from build123d import *

# Parameters (mm, degrees)
SKETCH2_R           = 2
BOSS_EXTRUDE2_DEPTH = 3.175


with BuildPart() as part:
    # Sketch2 → Boss-Extrude2 (new body)
    with BuildSketch(Plane.XY):
        with BuildLine():
            ThreePointArc((9.456794765, 7.302125235), (10.51328966, 8.920913041), (10.82870315, 10.828049574))
            ThreePointArc((10.82870315, 10.828049574), (8.921045244, 10.513465667), (7.301533296, 9.457386704))
            ThreePointArc((7.301533296, 9.457386704), (5.308889045, 9.194845217), (4.539183834, 11.051485471))
            ThreePointArc((4.539183834, 11.051485471), (4.64471403, 12.981928422), (3.964051405, 14.791471183))
            ThreePointArc((3.964051405, 14.791471183), (2.469674584, 13.565372247), (1.59532555, 11.841424903))
            ThreePointArc((1.59532555, 11.841424903), (0.000409384, 10.617090374), (-1.594506782, 11.841424903))
            ThreePointArc((-1.594506782, 11.841424903), (-2.468043552, 13.565085875), (-3.961395494, 14.791451895))
            ThreePointArc((-3.961395494, 14.791451895), (-4.64300424, 12.982116437), (-4.538365066, 11.051485471))
            ThreePointArc((-4.538365066, 11.051485471), (-5.308070277, 9.194845217), (-7.300714528, 9.457386704))
            ThreePointArc((-7.300714528, 9.457386704), (-8.919846484, 10.513683908), (-10.827230806, 10.82870315))
            ThreePointArc((-10.827230806, 10.82870315), (-10.512252617, 8.921293027), (-9.455975997, 7.302125235))
            ThreePointArc((-9.455975997, 7.302125235), (-9.19343451, 5.309480984), (-11.050074764, 4.539775774))
            ThreePointArc((-11.050074764, 4.539775774), (-12.980517715, 4.64530597), (-14.790060475, 3.964643344))
            ThreePointArc((-14.790060475, 3.964643344), (-13.56396154, 2.470266524), (-11.840014195, 1.595917489))
            ThreePointArc((-11.840014195, 1.595917489), (-10.615679667, 0.001001323), (-11.840014195, -1.593914842))
            ThreePointArc((-11.840014195, -1.593914842), (-13.563675168, -2.467451613), (-14.790041187, -3.960803554))
            ThreePointArc((-14.790041187, -3.960803554), (-12.980705729, -4.6424123), (-11.050074764, -4.537773127))
            ThreePointArc((-11.050074764, -4.537773127), (-9.19343451, -5.307478337), (-9.455975997, -7.300122588))
            ThreePointArc((-9.455975997, -7.300122588), (-10.512273201, -8.919254544), (-10.827292443, -10.826638866))
            ThreePointArc((-10.827292443, -10.826638866), (-8.91988232, -10.511660678), (-7.300714528, -9.455384057))
            ThreePointArc((-7.300714528, -9.455384057), (-5.308070277, -9.19284257), (-4.538365066, -11.049482824))
            ThreePointArc((-4.538365066, -11.049482824), (-4.643895262, -12.979925775), (-3.963232637, -14.789468536))
            ThreePointArc((-3.963232637, -14.789468536), (-2.468855816, -13.5633696), (-1.594506782, -11.839422256))
            ThreePointArc((-1.594506782, -11.839422256), (0.000409384, -10.615087727), (1.59532555, -11.839422256))
            ThreePointArc((1.59532555, -11.839422256), (2.46886232, -13.563083228), (3.962214262, -14.789449248))
            ThreePointArc((3.962214262, -14.789449248), (4.643823008, -12.98011379), (4.539183834, -11.049482824))
            ThreePointArc((4.539183834, -11.049482824), (5.308889045, -9.19284257), (7.301533296, -9.455384057))
            ThreePointArc((7.301533296, -9.455384057), (8.920665252, -10.511681261), (10.828049574, -10.826700503))
            ThreePointArc((10.828049574, -10.826700503), (10.513071385, -8.91929038), (9.456794765, -7.300122588))
            ThreePointArc((9.456794765, -7.300122588), (9.194253278, -5.307478337), (11.050893532, -4.537773127))
            ThreePointArc((11.050893532, -4.537773127), (12.981336483, -4.643303323), (14.790879243, -3.962640697))
            ThreePointArc((14.790879243, -3.962640697), (13.564780308, -2.468263877), (11.840832964, -1.593914842))
            ThreePointArc((11.840832964, -1.593914842), (10.617899153, 0.000932392), (11.841424903, 1.59532555))
            ThreePointArc((11.841424903, 1.59532555), (13.565085875, 2.46886232), (14.791451895, 3.962214262))
            ThreePointArc((14.791451895, 3.962214262), (12.982116437, 4.643823008), (11.051485471, 4.539183834))
            ThreePointArc((11.051485471, 4.539183834), (9.193282623, 5.308357949), (9.456794765, 7.302125235))
        make_face()
        Circle(SKETCH2_R, mode=Mode.SUBTRACT)
    extrude(amount=BOSS_EXTRUDE2_DEPTH)


solid = part.part
Verification items for the finished model (mm, model axes). A direction names the side the tool comes from. Give positions to 0.01 mm unless a question says otherwise; leave off trailing zeros. Write each loop counter-clockwise with the first axis right and the second up, starting at its lowest first coordinate (ties: lowest second). Pieces come first, ordered by that corner, then holes. Notation, with made-up numbers: M 33,72.5 L 58,72.5 A13 ccw 58,88.5 Z; hole C -21.5,84.5 d2. An arc over 180 degrees is marked long. Put each result on its own line as item: value. Start each with the question number.
1. Section check B-B (x = 0). Record the cut outline in (y, z) (3 decimals), and give its area (3 significant figures).
2. Section check D-D (x = 8). Record the cut outline in (y, z) (3 decimals), and give its area (3 significant figures).
3. Section check A-A (y = 0). Record the cut outline in (x, z) (3 decimals), and give its area (3 significant figures).
4. Set-up check for faces 1 (the face through (2.45, -13.54, 1.57)), 2 (the face through (-13.54, -2.45, 1.57)), 3 (the face through (-5.33, -9.18, 1.57)), 4 (the face through (13.59, -2.49, 1.57)): record each of +Z, -Z, +X, -X, +Y, -Y from which the full face is reachable in a straight line by a thin tool's end or side.
5. Draft check along X on faces 5 (the face through (0, -2, 2)), 6 (the face through (-4.65, -12.95, 1.57)), 7 (the face through (4.64, -13.01, 1.57)). Enter one of: +X half, -X half, draft (parallel to the pull), parting line (faces both ways), or undercut.
6. Go/stop test with flat-tipped pins: pin 1 Ø1 at (y, z) = (7, 2.5) entering from +X; pin 2 Ø5 at (x, y) = (0, 0) entering from +Z (3 decimals); pin 3 Ø1.5 at (x, z) = (3, 2.5) entering from -Y. Record where each tip stops, or that it passes through.
7. Scan lines: line 1 along Y through (x, z) = (0, 1.3); line 2 along Y through (x, z) = (12.5, 2.6); line 3 along X through (y, z) = (-0.25, 1.05). Record each from-to range of solid material in increasing order. Write a range as [from, to].
8. Section check C-C (y = 10). Record the cut outline in (x, z) (3 decimals).
Answer list:
1. outline: M -10.615,0 L -2,0 L -2,3.175 L -10.615,3.175 Z; M 2,0 L 10.617,0 L 10.617,3.175 L 2,3.175 Z
1. area: 54.7 mm2
2. outline: M -10.03,0 L 10.032,0 L 10.032,3.175 L -10.03,3.175 Z
2. area: 63.7 mm2
3. outline: M -10.616,0 L -2,0 L -2,3.175 L -10.616,3.175 Z; M 2,0 L 10.618,0 L 10.618,3.175 L 2,3.175 Z
3. area: 54.7 mm2
4. face 1: +Z, -Z, -Y
4. face 2: +Z, -Z, -X
4. face 3: +Z, -Z
4. face 4: +Z, -Z, +X
5. face 5: undercut
5. face 6: -X half
5. face 7: +X half
6. pin 1: x = 9.64
6. pin 2: z = 3.175
6. pin 3: y = -14.67
7. line 1: [-10.62, -2], [2, 10.62]
7. line 2: [-4.69, -1.82], [1.83, 4.69]
7. line 3: [-10.63, -1.98], [1.98, 10.64]
8. outline: M -10.79,0 L -7.952,0 L -7.952,3.175 L -10.79,3.175 Z; M -4.605,0 L 4.606,0 L 4.606,3.175 L -4.605,3.175 Z; M 7.953,0 L 10.791,0 L 10.791,3.175 L 7.953,3.175 Z
